CAD build for the part. Positions are in the model's coordinates, mm. Coordinates: 2 decimals unless noted, no trailing zeros. Loops run counter-clockwise (first coordinate to the right, second up) from the corner with the lowest first, then second, coordinate; pieces in that order, holes last. Notation, with made-up numbers: (-33.5, 84) -> (24.5, 84) arc R27 ccw to (24.5, 112) -> close; hole circle Ø6 at (11, -31.5). An arc over 180 degrees is marked (long way). Return JSON: item names as keys, results as strings. Group by question number.
(1) Probe L1, parallel to Y at x = -109.7, z = 2.1; L2, parallel to Y at x = -133.5, z = 2.3; L3, parallel to Y at x = -101, z = 2.6. List the from-to ranges inside material, lowest first.
(2) Saw through at C-C on z = 1.3. Give the number of separate pieces and of enclosed holes in the cut face, then the cut area to 3 significant figures.
(3) Saw through at D-D on x = -97.5. Write the cut outline in (y, z) (3 decimals), then the cut area to 3 significant figures.
(4) Flat gauge pin, fed straight in: pin 1 Ø1 at (x, z) = (-91.5, 1.5) entering from -Y. Where does the tip first touch, or does it go through?
(5) Saw through at A-A on x = -114. Write the cut outline in (y, z) (3 decimals), then the cut area to 3 significant figures.
(6) Saw through at B-B on x = -122.4. Write the cut outline in (y, z) (3 decimals).
```python
from build123d import *

# Parameters (mm, degrees)
SKETCH2_R           = 14.351
SKETCH2_R_2         = 2.5527
SKETCH2_R_3         = 3.175
BOSS_EXTRUDE1_DEPTH = 3.175


with BuildPart() as part:
    # Sketch2 → Boss-Extrude1 (new body)
    with BuildSketch(Plane.XY):
        with BuildLine():
            Line((-139.7, 154.014440652), (-139.7, 30))
            ThreePointArc((-139.7, 30), (-111.788337372, 0.072774151), (-79.990743532, 25.833457055))
            Line((-79.990743532, 25.833457055), (-68.399622728, 108.48317056))
            ThreePointArc((-68.399622728, 108.48317056), (-70.065229263, 119.947916289), (-77.629824678, 128.72239838))
            Line((-77.629824678, 128.72239838), (-127.122524146, 160.845515232))
            ThreePointArc((-127.122524146, 160.845515232), (-135.443000435, 161.170844756), (-139.7, 154.014440652))
        make_face()
        with Locations((-88.9, 111.358224077)):
            Circle(SKETCH2_R, mode=Mode.SUBTRACT)
        with Locations((-109.7, 55.4)):
            Circle(SKETCH2_R_2, mode=Mode.SUBTRACT)
        with Locations((-97, 51.997045256)):
            Circle(SKETCH2_R_2, mode=Mode.SUBTRACT)
        with Locations((-87.702954744, 42.7)):
            Circle(SKETCH2_R_2, mode=Mode.SUBTRACT)
        with Locations((-84.3, 30)):
            Circle(SKETCH2_R_2, mode=Mode.SUBTRACT)
        with Locations((-87.702954744, 17.3)):
            Circle(SKETCH2_R_2, mode=Mode.SUBTRACT)
        with Locations((-97, 8.002954744)):
            Circle(SKETCH2_R_2, mode=Mode.SUBTRACT)
        with Locations((-109.7, 4.6)):
            Circle(SKETCH2_R_2, mode=Mode.SUBTRACT)
        with Locations((-122.4, 8.002954744)):
            Circle(SKETCH2_R_2, mode=Mode.SUBTRACT)
        with Locations((-131.697045256, 17.3)):
            Circle(SKETCH2_R_2, mode=Mode.SUBTRACT)
        with Locations((-135.1, 30)):
            Circle(SKETCH2_R_2, mode=Mode.SUBTRACT)
        with Locations((-131.697045256, 42.7)):
            Circle(SKETCH2_R_2, mode=Mode.SUBTRACT)
        with Locations((-122.4, 51.997045256)):
            Circle(SKETCH2_R_2, mode=Mode.SUBTRACT)
        with Locations((-109.7, 30)):
            Circle(SKETCH2_R, mode=Mode.SUBTRACT)
        with Locations((-131.556216575, 68.702007502)):
            Circle(SKETCH2_R_3, mode=Mode.SUBTRACT)
        with Locations((-131.556216575, 154.014440652)):
            Circle(SKETCH2_R_3, mode=Mode.SUBTRACT)
    extrude(amount=BOSS_EXTRUDE1_DEPTH)


solid = part.part
```
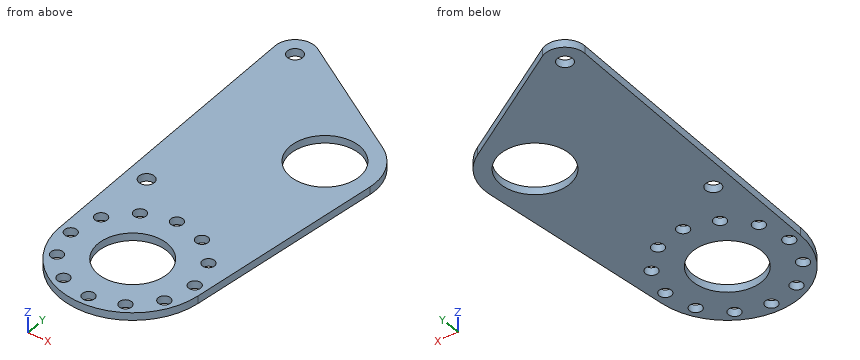
Geometry results:
{
 "1": {"L1": "0 to 2.05, 7.15 to 15.65, 44.35 to 52.85, 57.95 to 149.54", "L2": "11.74 to 15.49, 19.11 to 28.01, 31.99 to 40.89, 44.51 to 66.19, 71.21 to 151.5, 156.52 to 161.92", "L3": "1.29 to 18.59, 41.41 to 103.64, 119.07 to 143.89"},
 "2": {"separate pieces": "1", "enclosed holes": "16", "area": "7,570 mm²"},
 "3": {"outline": "(2.593, 0) -> (5.5, 0) -> (5.5, 3.175) -> (2.593, 3.175) -> close; (10.506, 0) -> (22.443, 0) -> (22.443, 3.175) -> (10.506, 3.175) -> close; (37.557, 0) -> (49.494, 0) -> (49.494, 3.175) -> (37.557, 3.175) -> close; (54.5, 0) -> (99.869, 0) -> (99.869, 3.175) -> (54.5, 3.175) -> close; (122.847, 0) -> (141.619, 0) -> (141.619, 3.175) -> (122.847, 3.175) -> close", "area": "289 mm²"},
 "4": {"pin 1": "y = 5.78"},
 "5": {"outline": "(0.31, 0) -> (16.308, 0) -> (16.308, 3.175) -> (0.31, 3.175) -> close; (43.692, 0) -> (152.328, 0) -> (152.328, 3.175) -> (43.692, 3.175) -> close", "area": "396 mm²"},
 "6": {"outline": "(2.821, 0) -> (5.45, 0) -> (5.45, 3.175) -> (2.821, 3.175) -> close; (10.556, 0) -> (23.317, 0) -> (23.317, 3.175) -> (10.556, 3.175) -> close; (36.683, 0) -> (49.444, 0) -> (49.444, 3.175) -> (36.683, 3.175) -> close; (54.55, 0) -> (157.78, 0) -> (157.78, 3.175) -> (54.55, 3.175) -> close"}
}
